For this review, use the dimensioned drawing (mm, ordinates from the lowest corner) and the shaded views. A direction names the side the tool comes from. Coordinates: 2 decimals unless noted, no trailing zeros. Loops run counter-clockwise (first coordinate to the right, second up) from the corner with the lowest first, then second, coordinate; pieces in that order, holes last. Notation, with made-up numbers: (65, 65) -> (74, 65) arc R30 cw to (74, 94) -> close; hole circle Ø9 at (28.5, 81.5). An arc over 180 degrees is marked (long way). Answer as a JSON object with one key per item and string values.
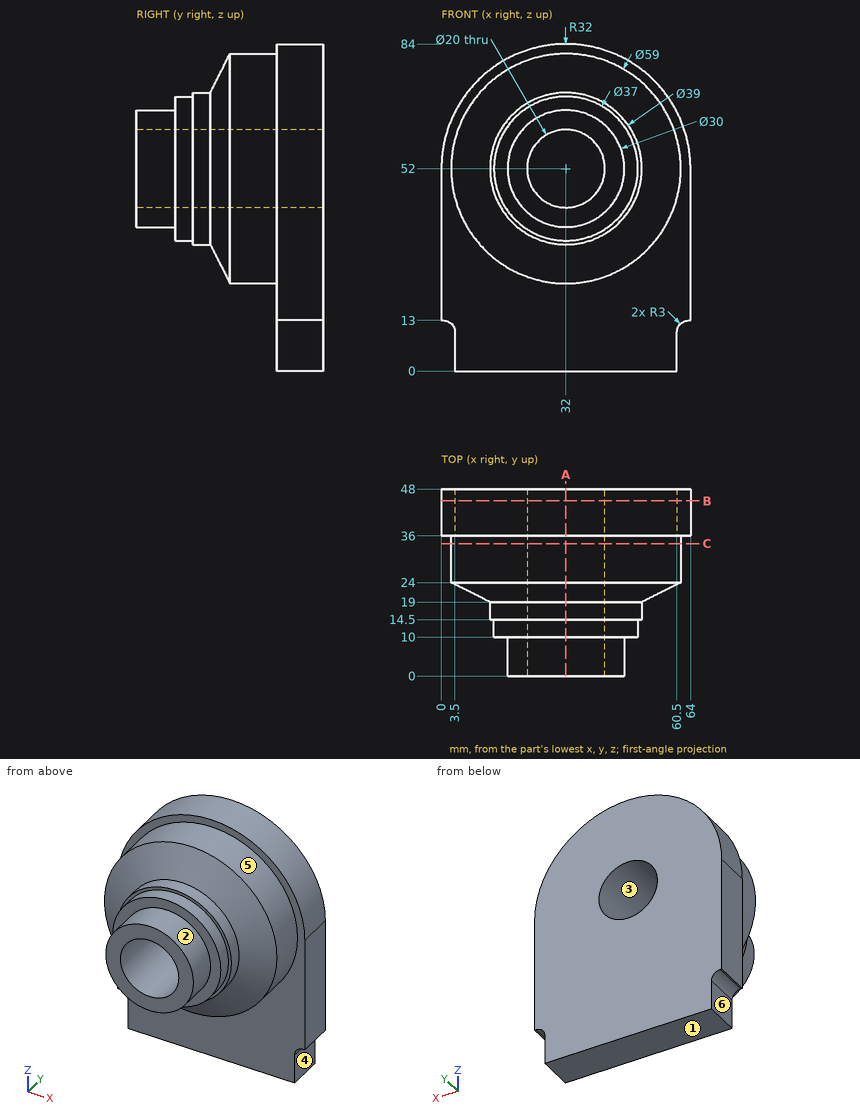
1) Add section C-C, the plane y = 34. Give the boundary of the cut face in (x, z), and give its area (3 significant figures).
Completed:
{"outline": "circle Ø59 at (32, 52); hole circle Ø20 at (32, 52)", "area": "2,420 mm²"}
2) Add section B-B, the plane y = 45. Give the boundary of the cut face in (x, z).
Completed:
{"outline": "(0, 13) -> (0.5, 13) arc R3 cw to (3.5, 10) -> (3.5, 0) -> (60.5, 0) -> (60.5, 10) arc R3 cw to (63.5, 13) -> (64, 13) -> (64, 52) arc R32 ccw to (0, 52) -> close; hole circle Ø20 at (32, 52)"}
3) Add section A-A, the plane x = 32. Give the boundary of the cut face in (y, z), and give its area (3 significant figures).
Completed:
{"outline": "(0, 37) -> (10, 37) -> (10, 33.5) -> (14.5, 33.5) -> (14.5, 32.5) -> (19, 32.5) -> (24, 22.5) -> (36, 22.5) -> (36, 0) -> (48, 0) -> (48, 42) -> (0, 42) -> close; (0, 62) -> (48, 62) -> (48, 84) -> (36, 84) -> (36, 81.5) -> (24, 81.5) -> (19, 71.5) -> (14.5, 71.5) -> (14.5, 70.5) -> (10, 70.5) -> (10, 67) -> (0, 67) -> close", "area": "1,640 mm²"}
4) For the marked faces 4, 5 and 6, list the 3-axis set-ups (+Z, -Z, +X, -X, +Y, -Y) from which the entire face can be reached by the end or side of a thin tool; tool diameter is ignored.
Completed:
{"face 4": "-Z, +X, +Y, -Y", "face 5": "-Y", "face 6": "-Z, -X, +Y, -Y"}
5) The part is to be moulded in two halves that separate along X. For the marked faces 1, 2 and 3, say which applies: pulls with the +X half, pulls with the -X half, needs draft (parallel to the pull), parting line crosses it, or undercut.
Completed:
{"face 1": "needs draft", "face 2": "parting line crosses it", "face 3": "undercut"}
6) Wall thickness on probe 1 along Z at (x, y) = (32, 11); probe 2 along Z at (x, y) = (32, 27); probe 3 along X at (y, z) = (40.5, 6.5): over which ranges is each line inside the solid? List them lowest first.
Completed:
{"probe 1": "33.5 to 42, 62 to 70.5", "probe 2": "22.5 to 42, 62 to 81.5", "probe 3": "3.5 to 60.5"}
7) Clearance check with flat-ended pins moving along their axes: pin 1 Ø6 at (x, z) = (41, 72.5) entering from -Y; pin 2 Ø10 at (y, z) = (9, 75.5) entering from -X; pin 3 Ø5 at (x, y) = (37, 11.5) entering from +Z; pin 4 Ø4 at (y, z) = (22, 44.5) entering from +X. State where each tip first meets the part, or that it passes through.
Completed:
{"pin 1": "y = 14.5", "pin 2": "through", "pin 3": "z = 70.33", "pin 4": "x = 60.56"}
